```python
from build123d import *

# Parameters (mm, degrees)
F0_W     = 762
F0_H     = 609.6
F1_DEPTH = 876.3
F2_W     = 2.54
F2_H     = 609.6
F3_DEPTH = 76.2
F4_W     = 762
F4_H     = 25.4
F4_H_2   = 609.6
F5_DEPTH = 25.4
F6_W     = 508
F6_H     = 355.6
F7_DEPTH = 762


with BuildPart() as f1:
    # F0 (on Top) → F1 (new body)
    with BuildSketch(Plane.XY):
        Rectangle(F0_W, F0_H)
    extrude(amount=F1_DEPTH)

    # F2 (on face) → F3 (cut)
    with BuildSketch(Plane.XZ.offset(304.8)):
        Polygon((-381, 88.9), (-381, 0), (381, 0), (381, 88.9), (1.27, 88.9), (-1.27, 88.9), align=None)
        Polygon((-381, 701.04), (-381, 698.5), (-1.27, 698.5), (1.27, 698.5), (381, 698.5), (381, 701.04), align=None)
        with Locations((0, 393.7)):
            Rectangle(F2_W, F2_H)
    extrude(amount=-F3_DEPTH, mode=Mode.SUBTRACT)

    # F4 (on face) → F5 (join)
    with BuildSketch(Plane.XY.offset(876.3)):
        with Locations((0, -317.5)):
            Rectangle(F4_W, F4_H)
        Rectangle(F4_W, F4_H_2)
    extrude(amount=-F5_DEPTH)

    # F6 (on face) → F7 (cut)
    with BuildSketch(Plane(origin=(0, 0, 0), x_dir=(1, 0, 0), z_dir=(0, 0, -1))):
        Rectangle(F6_W, F6_H)
    extrude(amount=-F7_DEPTH, mode=Mode.SUBTRACT)


solid = f1.part
```
Could you check a few things on this model? Use its own coordinates, in mm. A direction names the side the tool comes from. Give positions to 0.01 mm unless a question says otherwise; leave off trailing zeros. Write each loop counter-clockwise with the first axis right and the second up, starting at its lowest first coordinate (ties: lowest second). Pieces come first, ordered by that corner, then holes. Notation, with made-up numbers: (-10, -21.5) -> (14, -21.5) arc R10 cw to (14, -16.5) -> close; hole circle Ø8 at (11.25, 85). An arc over 180 degrees is marked (long way). Write each question's results on one line, items separated by ' | '.
1. I want a section at A-A, the plane y = -74. Write out the boundary of the cut face in (x, z), then the cut area to 3 significant figures.
Check sheet entries:
outline: (-381, 0) -> (-254, 0) -> (-254, 762) -> (254, 762) -> (254, 0) -> (381, 0) -> (381, 876.3) -> (-381, 876.3) -> close | area: 281,000 mm²
2. I want a section at B-B, the plane z = 640. Write out the boundary of the cut face in (x, y).
Check sheet entries:
outline: (-381, -304.8) -> (-1.27, -304.8) -> (-1.27, -228.6) -> (1.27, -228.6) -> (1.27, -304.8) -> (381, -304.8) -> (381, 304.8) -> (-381, 304.8) -> close; hole (-254, -177.8) -> (254, -177.8) -> (254, 177.8) -> (-254, 177.8) -> close
3. I need wall thicknesses on L1, parallel to Y at x = 60.5, z = 705; L2, parallel to X at y = -104.5, z = 114; L3, parallel to Z at x = -346, y = -250.5. Which ranges of each line are inside material? Lowest first, please.
Check sheet entries:
L1: y = -304.8 to -177.8, 177.8 to 304.8 | L2: x = -381 to -254, 254 to 381 | L3: z = 88.9 to 698.5, 701.04 to 876.3
4. Will these pins go through, and if not, where does the flat tip stop? pin 1 Ø3 at (x, y) = (-150.5, 189.5) entering from -Z; pin 2 Ø7.5 at (x, y) = (-79.5, -313) entering from -Z; pin 3 Ø6 at (x, z) = (109, 122) entering from -Y.
Check sheet entries:
pin 1: stops at z = 0 | pin 2: stops at z = 850.9 | pin 3: stops at y = -304.8
5. If we mould it in two halves opening along Z, with no side actions, what happens to faces 5 (the flat face through (-194, -267, 698.5)), 6 (the flat face through (-188, -267, 88.9)), 7 (the flat face through (-254, 2, 376))? For each: released by +Z, released by -Z, zero draft, split by the parting line, or undercut.
Check sheet entries:
face 5: undercut | face 6: released by -Z | face 7: zero draft
6. I want a section at C-C, the plane x = 235.5. Write out the boundary of the cut face in (y, z).
Check sheet entries:
outline: (-330.2, 850.9) -> (-304.8, 850.9) -> (-304.8, 701.04) -> (-228.6, 701.04) -> (-228.6, 698.5) -> (-304.8, 698.5) -> (-304.8, 88.9) -> (-228.6, 88.9) -> (-228.6, 0) -> (-177.8, 0) -> (-177.8, 762) -> (177.8, 762) -> (177.8, 0) -> (304.8, 0) -> (304.8, 876.3) -> (-330.2, 876.3) -> close
7. On a 3-axis mill with a long thin cutter (end or side, diameter ignored), from which of +Z, -Z, +X, -X, +Y, -Y can I reach the whole of each face in a straight line? I mean faces 1 (the flat face through (-194, -304.8, 389)), 2 (the flat face through (-4, -177.8, 376)), 3 (the flat face through (-1.27, -267, 389)), 4 (the flat face through (188, -267, 698.5)). Say none if no direction works.
Check sheet entries:
face 1: -Z, +X, -X, -Y | face 2: -Z | face 3: -Z, -Y | face 4: +X, -X, -Y
